Can you work these out from the model? Positions are in its coordinate system, mm. A direction names the side the tool comes from. Round coordinates to 2 decimals unless told otherwise and drop trailing zeros. Order: outer loops, then holes, each group sorted by start corner. A loop starts at its lowest first (then second) coordinate and runs counter-clockwise, first axis right, second up. Notation, with made-up numbers: (9.25, -29) - (24.25, -29) arc R20 cw to (24.25, -4) - close; hole circle Ø2 at (60, 23.5). An arc over 180 degrees is marked (long way). Write item = value, one per line.
from build123d import *

# Parameters (mm, degrees)
BOSS_EXTRUDE2_DEPTH     = 45
BOSS_EXTRUDE4_START     = -24
SKETCH2_R               = 12.5
BOSS_EXTRUDE4_DEPTH     = 10
BOSS_EXTRUDE6_START     = 10
SKETCH3_W               = 25
SKETCH3_H               = 40
BOSS_EXTRUDE6_DEPTH     = 25
CUT_EXTRUDE1_DEPTH      = 46.0000001
CUT_EXTRUDE1_DEPTH_BACK = 20


with BuildPart() as part:
    # Sketch1 → Boss-Extrude2 (new body)
    with BuildSketch(Plane(origin=(0, 0, 0), x_dir=(1, 0, 0), z_dir=(0, 1, 0))):
        with BuildLine():
            ThreePointArc((-2.801227604, 12.840197836), (-3.388966753, 13.401826964), (-3.866028841, 14.06006427))
            ThreePointArc((-3.866028841, 14.06006427), (-3.636455498, 13.666793472), (-3.413425605, 13.269775202))
            Line((-3.413425605, 13.269775202), (-2.801227604, 12.840197836))
        make_face()
        with BuildLine():
            Line((-4.349767454, 17.506911707), (-12.023106204, 22.731382677))
            ThreePointArc((-12.023106204, 22.731382677), (-7.469700948, 18.842428715), (-3.866028841, 14.06006427))
            ThreePointArc((-3.866028841, 14.06006427), (-4.454774574, 15.734806542), (-4.349767454, 17.506911707))
        make_face()
        with BuildLine():
            Line((-0.844194207, 15.120106399), (-4.349767454, 17.506911707))
            ThreePointArc((-4.349767454, 17.506911707), (-4.454774574, 15.734806542), (-3.866028841, 14.06006427))
            ThreePointArc((-3.866028841, 14.06006427), (-3.388966753, 13.401826964), (-2.801227604, 12.840197836))
            Line((-2.801227604, 12.840197836), (-2.357112674, 12.528563819))
            ThreePointArc((-2.357112674, 12.528563819), (0, 11.861568788), (2.357112674, 12.528563819))
            Line((2.357112674, 12.528563819), (2.801227604, 12.840197836))
            ThreePointArc((2.801227604, 12.840197836), (3.388966727, 13.401826933), (3.8660288, 14.0600642))
            ThreePointArc((3.8660288, 14.0600642), (4.337450172, 15.167351949), (4.498431212, 16.36))
            ThreePointArc((4.498431212, 16.36), (4.461110458, 16.93825327), (4.349767454, 17.506911707))
            Line((4.349767454, 17.506911707), (0.844194207, 15.120106399))
            ThreePointArc((0.844194207, 15.120106399), (0, 14.86), (-0.844194207, 15.120106399))
        make_face()
        with BuildLine():
            Line((12.023106204, 22.731382677), (4.349767454, 17.506911707))
            ThreePointArc((4.349767454, 17.506911707), (4.461110458, 16.93825327), (4.498431212, 16.36))
            ThreePointArc((4.498431212, 16.36), (4.337450172, 15.167351949), (3.8660288, 14.0600642))
            ThreePointArc((3.8660288, 14.0600642), (7.46970092, 18.842428685), (12.023106204, 22.731382677))
        make_face()
        with BuildLine():
            Line((2.801227604, 12.840197836), (3.413425605, 13.269775202))
            ThreePointArc((3.413425605, 13.269775202), (3.636455478, 13.666793437), (3.8660288, 14.0600642))
            ThreePointArc((3.8660288, 14.0600642), (3.388966727, 13.401826933), (2.801227604, 12.840197836))
        make_face()
        with BuildLine():
            Line((52.2, 0), (55, 0))
            ThreePointArc((55, 0), (40.357593488, 24.309098908), (12.023106204, 22.731382677))
            ThreePointArc((12.023106204, 22.731382677), (7.46970092, 18.842428685), (3.8660288, 14.0600642))
            ThreePointArc((3.8660288, 14.0600642), (3.636455478, 13.666793437), (3.413425605, 13.269775202))
            Line((3.413425605, 13.269775202), (13.028813696, 20.016862066))
            ThreePointArc((13.028813696, 20.016862066), (13.312464415, 20.218897943), (13.59893539, 20.416914623))
            ThreePointArc((13.59893539, 20.416914623), (39.048456696, 21.833990655), (52.2, 0))
        make_face()
        with BuildLine():
            ThreePointArc((-12.023106204, 22.731382677), (-40.357593488, 24.309098908), (-55, 0))
            Line((-55, 0), (-52.2, 0))
            ThreePointArc((-52.2, 0), (-39.048456696, 21.833990655), (-13.59893539, 20.416914623))
            ThreePointArc((-13.59893539, 20.416914623), (-13.312464415, 20.218897943), (-13.028813696, 20.016862066))
            Line((-13.028813696, 20.016862066), (-3.413425605, 13.269775202))
            ThreePointArc((-3.413425605, 13.269775202), (-3.636455498, 13.666793472), (-3.866028841, 14.06006427))
            ThreePointArc((-3.866028841, 14.06006427), (-7.469700948, 18.842428715), (-12.023106204, 22.731382677))
        make_face()
    extrude(amount=BOSS_EXTRUDE2_DEPTH)

    # Sketch2 → Boss-Extrude4 (add)
    with BuildSketch(Plane.XY.offset(BOSS_EXTRUDE4_START)):
        with Locations((-27.5, 22.5)):
            Circle(SKETCH2_R)
        with Locations((27.5, 22.5)):
            Circle(SKETCH2_R)
    extrude(amount=-BOSS_EXTRUDE4_DEPTH)

    # Sketch3 → Boss-Extrude6 (add)
    with BuildSketch(Plane.XY.offset(BOSS_EXTRUDE6_START)):
        with Locations((0, 25)):
            Rectangle(SKETCH3_W, SKETCH3_H)
    extrude(amount=-BOSS_EXTRUDE6_DEPTH)

    # Sketch5 → Cut-Extrude1 (cut, two sides)
    with BuildSketch(Plane(origin=(0, 0, 0), x_dir=(1, 0, 0), z_dir=(0, 1, 0))) as cut_extrude1_sk:
        Polygon((-9.94603189, 10), (9.94603189, 10), (9.94603189, 5), (4.94603189, 5), (4.94603189, 0), (9.94603189, 0), (9.94603189, -5), (-9.94603189, -5), (-9.94603189, 0), (-4.94603189, 0), (-4.94603189, 5), (-9.94603189, 5), align=None)
    extrude(amount=CUT_EXTRUDE1_DEPTH, mode=Mode.SUBTRACT)
    extrude(cut_extrude1_sk.sketch, amount=-CUT_EXTRUDE1_DEPTH_BACK, mode=Mode.SUBTRACT)


solid = part.part
(1) Will these pins go through, and if not, where does the flat tip stop? P1, Ø3.5, axis at x = -26.5, y = 24, coming from the +Z side; P2, Ø4, axis at x = 13.5, z = -0.5, coming from the -Y side; P3, Ø12, axis at y = 13.5, z = -19.5, coming from the +X side.
Computed:
P1 = -24
P2 = 5
P3 = 51.46
(2) On a 3-axis mill with a long thin cutter (end or side, diameter ignored), from which of +Z, -Z, +X, -X, +Y, -Y can I reach the whole of each face in a straight line? I mean faces 1 (the face through (46.097, 22.185, -20.259)), 2 (the face through (27, 23, -24)), 3 (the face through (-9.946, 25, 3)). Say none if no direction works.
Computed:
face_1 = -Z
face_2 = +Z, +Y, -Y
face_3 = +Y, -Y
(3) If we section it at D-D (z = -21.5): Write out the boundary of the cut face in (x, y).
Computed:
outline = (-44.65, 0) - (-39.66, 0) - (-39.66, 45) - (-44.65, 45) - close; (-15.34, 0) - (-10.21, 0) - (-10.21, 45) - (-15.34, 45) - close; (10.21, 0) - (15.34, 0) - (15.34, 45) - (10.21, 45) - close; (39.66, 0) - (44.65, 0) - (44.65, 45) - (39.66, 45) - close
(4) If we section it at B-B (x = -27.5): Write out the boundary of the cut face in (y, z).
Computed:
outline = (0, -27.5) - (10, -27.5) - (10, -34) - (35, -34) - (35, -27.5) - (45, -27.5) - (45, -24.7) - (35, -24.7) - (35, -24) - (10, -24) - (10, -24.7) - (0, -24.7) - close
(5) If I drill on line 1 (X direction, y = 8.5, z = 4); line 2 (X direction, y = 6.5, z = -20); line 3 (X direction, y = 30, z = -7), over which ranges is the centre line in solid material (lowest first)? Write a range as from..to.
Computed:
line_1 = -12.5..-9.95, 9.95..12.5
line_2 = -46.37..-41.99, -13..-8.01, 8.01..13, 41.99..46.37
line_3 = -54.09..-51.19, -12.5..-9.95, 9.95..12.5, 51.19..54.09
(6) If we section it at C-C (z = -29): Write out the boundary of the cut face in (x, y).
Computed:
outline = circle Ø25 at (-27.5, 22.5); circle Ø25 at (27.5, 22.5)
(7) Thinking about a two-plate mould opening in X: for faces 4 (the face through (-0.03, 2.46, -11.86)), 5 (the face through (-7, 25, 0)), 6 (the face through (27, 23, -34)), which applies, +X half, -X half, draft (parallel to the pull), parting line (faces both ways), or undercut?
Computed:
face_4 = undercut
face_5 = undercut
face_6 = draft
